from build123d import *

# Parameters (mm, degrees)
SKETCH1_R           = 1.5
BOSS_EXTRUDE1_DEPTH = 9
SKETCH4_R           = 1.5
BOSS_EXTRUDE4_DEPTH = 23
SKETCH5_R           = 1.5
BOSS_EXTRUDE6_DEPTH = 8
SKETCH2_R           = 11
SKETCH2_R_2         = 4.5
BOSS_EXTRUDE2_DEPTH = 2
SKETCH3_R           = 2.5
BOSS_EXTRUDE3_DEPTH = 24
CHAMFER1_SIZE       = 0.1


with BuildPart() as part:
    # Sketch1 → Boss-Extrude1 (new body)
    with BuildSketch(Plane(origin=(0, 0, 0), x_dir=(1, 0, 0), z_dir=(0, 1, 0))):
        Polygon((-15.5, -21.15), (15.5, -21.15), (21.15, -15.5), (21.15, 15.5), (15.5, 21.15), (-15.5, 21.15), (-21.15, 15.5), (-21.15, -15.5), align=None)
        with Locations((-15.5, 15.5)):
            Circle(SKETCH1_R, mode=Mode.SUBTRACT)
        with Locations((15.5, -15.5)):
            Circle(SKETCH1_R, mode=Mode.SUBTRACT)
        with Locations((15.5, 15.5)):
            Circle(SKETCH1_R, mode=Mode.SUBTRACT)
        with Locations((-15.5, -15.5)):
            Circle(SKETCH1_R, mode=Mode.SUBTRACT)
    extrude(amount=BOSS_EXTRUDE1_DEPTH)

    # Sketch4 → Boss-Extrude4 (add)
    with BuildSketch(Plane(origin=(0, 9, 0), x_dir=(1, 0, 0), z_dir=(0, 1, 0))):
        Polygon((13.478679656, 21.05), (-13.478679656, 21.05), (-21.05, 13.478679656), (-21.05, -13.478679656), (-13.478679656, -21.05), (13.478679656, -21.05), (21.05, -13.478679656), (21.05, 13.478679656), align=None)
        with Locations((-15.5, 15.5)):
            Circle(SKETCH4_R, mode=Mode.SUBTRACT)
        with Locations((15.5, 15.5)):
            Circle(SKETCH4_R, mode=Mode.SUBTRACT)
        with Locations((15.5, -15.5)):
            Circle(SKETCH4_R, mode=Mode.SUBTRACT)
        with Locations((-15.5, -15.5)):
            Circle(SKETCH4_R, mode=Mode.SUBTRACT)
    extrude(amount=BOSS_EXTRUDE4_DEPTH)

    # Sketch5 → Boss-Extrude6 (add)
    with BuildSketch(Plane(origin=(0, 32, 0), x_dir=(1, 0, 0), z_dir=(0, 1, 0))):
        Polygon((-15.5, 21.15), (-21.15, 15.5), (-21.15, -15.5), (-15.5, -21.15), (15.5, -21.15), (21.15, -15.5), (21.15, 15.5), (15.5, 21.15), align=None)
        with Locations((15.5, 15.5)):
            Circle(SKETCH5_R, mode=Mode.SUBTRACT)
        with Locations((-15.5, 15.5)):
            Circle(SKETCH5_R, mode=Mode.SUBTRACT)
        with Locations((-15.5, -15.5)):
            Circle(SKETCH5_R, mode=Mode.SUBTRACT)
        with Locations((15.5, -15.5)):
            Circle(SKETCH5_R, mode=Mode.SUBTRACT)
    extrude(amount=BOSS_EXTRUDE6_DEPTH)

    # Sketch2 → Boss-Extrude2 (add)
    with BuildSketch(Plane(origin=(0, 40, 0), x_dir=(1, 0, 0), z_dir=(0, 1, 0))):
        Circle(SKETCH2_R)
        Circle(SKETCH2_R_2, mode=Mode.SUBTRACT)
    extrude(amount=BOSS_EXTRUDE2_DEPTH)

    # Sketch3 → Boss-Extrude3 (add)
    with BuildSketch(Plane(origin=(0, 40, 0), x_dir=(1, 0, 0), z_dir=(0, 1, 0))):
        Circle(SKETCH3_R)
    extrude(amount=BOSS_EXTRUDE3_DEPTH)

    # Chamfer1
    chamfer1_edges = [part.edges().sort_by_distance(p)[0] for p in [
        (-21.15, 0, 0),
        (-18.325, 0, -18.325),
        (-11, 42, 0),
        (-11, 40, 0),
        (-4.5, 42, 0),
        (-2.5, 64, 0),
        (-17, 0, -15.5),
        (14, 0, 15.5),
        (14, 0, -15.5),
        (-17, 0, 15.5),
        (0, 40, -21.15),
        (-18.325, 40, -18.325),
        (-21.15, 40, 0),
        (-18.325, 40, 18.325),
        (0, 40, 21.15),
        (18.325, 40, 18.325),
        (21.15, 40, 0),
        (18.325, 40, -18.325),
        (0, 0, -21.15),
        (14, 40, -15.5),
        (18.325, 0, -18.325),
        (-17, 40, -15.5),
        (-17, 40, 15.5),
        (14, 40, 15.5),
        (21.15, 0, 0),
        (18.325, 0, 18.325),
        (0, 0, 21.15),
        (-18.325, 0, 18.325),
    ]]
    chamfer(chamfer1_edges, length=CHAMFER1_SIZE)


solid = part.part
Geometry: final body of the model. Coordinates: model frame, mm. A direction names the side the tool comes from. Round coordinates to 2 decimals unless told otherwise and drop trailing zeros. Write each loop counter-clockwise with the first axis right and the second up, starting at its lowest first coordinate (ties: lowest second). Pieces come first, ordered by that corner, then holes. Notation, with made-up numbers: M 62,-33.75 L 106,-33.75 A16 cw 106,-3.75 Z; hole C 22.25,-25.5 d1. An arc over 180 degrees is marked long. Write item = value, one per line.
Item 1: Section query C-C on y = 17. Return loops of the section in (x, z), then the cut area to 3 significant figures.
Findings:
outline = M -21.05,-13.48 L -13.48,-21.05 L 13.48,-21.05 L 21.05,-13.48 L 21.05,13.48 L 13.48,21.05 L -13.48,21.05 L -21.05,13.48 Z; hole C -15.5,-15.5 d3; hole C -15.5,15.5 d3; hole C 15.5,-15.5 d3; hole C 15.5,15.5 d3
area = 1,630 mm^2
Item 2: Pin query (flat end, axial travel): P1, Ø12.5, axis at x = -2, z = 5.5, coming from the +Y side; P2, Ø2.5, axis at x = -15.5, z = -15.5, coming from the +Y side; P3, Ø2, axis at y = 16, z = -2.5, coming from the -X side; P4, Ø11.5, axis at x = -1, y = 24, coming from the -Z side. Return the tip coordinate at first contact, or that it passes through.
Findings:
P1 = 64
P2 = through
P3 = -21.05
P4 = -21.05
Item 3: Pull-direction query (X, two-part tool) for faces 3 (the face through (-17, 19.72, -15.57)), 4 (the face through (18.29, 4.49, 18.36)), 5 (the face through (-17.21, 20.34, -17.32)); classes: pulls with the +X half, pulls with the -X half, needs draft (parallel to the pull), parting line crosses it, or undercut.
Findings:
face_3 = undercut
face_4 = pulls with the +X half
face_5 = pulls with the -X half
Item 4: Section query B-B on z = -18. Return loops of the section in (x, y), then the cut area to 3 significant figures.
Findings:
outline = M -18.65,0.1 L -18.51,0 L 18.51,0 L 18.65,0.1 L 18.65,9 L 16.53,9 L 16.53,32 L 18.65,32 L 18.65,39.9 L 18.51,40 L -18.51,40 L -18.65,39.9 L -18.65,32 L -16.53,32 L -16.53,9 L -18.65,9 Z
area = 1,390 mm^2
Item 5: Material intervals for line 1 along Z through (x, y) = (0, 41.25); line 2 along Z through (x, y) = (15.5, 10), sorted ascending. Write a range as [from, to].
Findings:
line_1 = [-11, -4.5], [-2.5, 2.5], [4.5, 11]
line_2 = [-19.03, -17], [-14, 14], [17, 19.03]
Item 6: Access query for faces 1 (the face through (0, 36, 21.15)), 2 (the face through (2, 40, 2)). Directions: +Z, -Z, +X, -X, +Y, -Y. A direction counts if a zero-diameter tool reaches every point of the face in a straight line with its end or side. Return the directions, or none.
Findings:
face_1 = +Z, +X, -X, +Y, -Y
face_2 = +Y
Item 7: Section query A-A on y = 34. Return loops of the section in (x, z), then the cut area to 3 significant figures.
Findings:
outline = M -21.15,-15.5 L -15.5,-21.15 L 15.5,-21.15 L 21.15,-15.5 L 21.15,15.5 L 15.5,21.15 L -15.5,21.15 L -21.15,15.5 Z; hole C -15.5,-15.5 d3; hole C -15.5,15.5 d3; hole C 15.5,-15.5 d3; hole C 15.5,15.5 d3
area = 1,700 mm^2
Item 8: Section query D-D on x = -18. Return loops of the section in (y, z).
Findings:
outline = M 0,-18.51 L 0.1,-18.65 L 9,-18.65 L 9,-16.53 L 32,-16.53 L 32,-18.65 L 39.9,-18.65 L 40,-18.51 L 40,18.51 L 39.9,18.65 L 32,18.65 L 32,16.53 L 9,16.53 L 9,18.65 L 0.1,18.65 L 0,18.51 Z
